Geometry check sheet. Reference: the model listing, model coordinates, mm. Coordinates: 2 decimals unless noted, no trailing zeros. Order: outer loops, then holes, each group sorted by start corner. A loop starts at its lowest first (then second) coordinate and runs counter-clockwise, first axis right, second up. Notation, with made-up numbers: (-13, 53.25) - (3, 53.25) arc R22 ccw to (3, 86.25) - close; hole circle Ø9 at (20, -18.75). An arc over 180 degrees is marked (long way). Use CSV: the item, a comma, the result in double quotes. Start each with the question number.
1) Depth check by flat-ended pin: P1, Ø4, axis at x = 5, y = 6, coming from the +Z side. Enter the tip coordinate at first touch or a pass-through.
2) Sectioned sample at B-B, the plane y = 6. Record the cut outline in (x, z).
3) Sectioned sample at C-C, the plane z = 8.75. Record the cut outline in (x, y).
4) Sectioned sample at D-D, the plane x = 7. Record the cut outline in (y, z), and give its area (3 significant figures).
5) Sectioned sample at A-A, the plane x = 5. Record the cut outline in (y, z), and give its area (3 significant figures).
6) Thickness scan on probe 1 along Y at (x, z) = (5, 2); probe 2 along Y at (x, z) = (5, 9.35); probe 3 along X at (y, z) = (14, 2.25). Record the ranges inside material, lowest first. Write a range as [from, to].
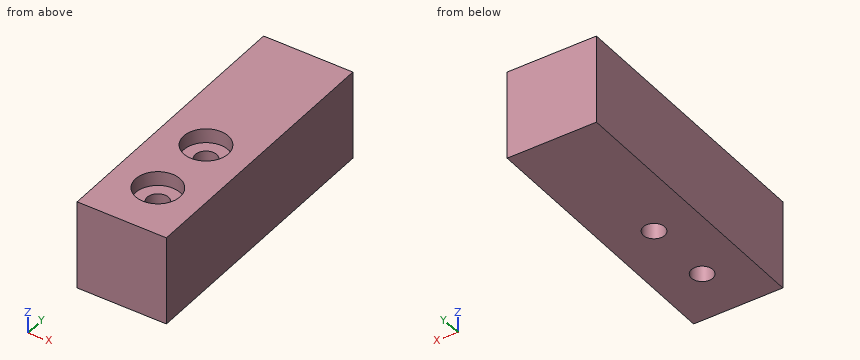
from build123d import *

# Parameters (mm, degrees)
SKETCH1_W                                = 10
SKETCH1_H                                = 31
BOSS_EXTRUDE1_DEPTH                      = 10
CBORE_FOR_M2_PAN_HEAD_SCREW1_D           = 2.4
CBORE_FOR_M2_PAN_HEAD_SCREW1_DEPTH       = 10
CBORE_FOR_M2_PAN_HEAD_SCREW1_CBORE_D     = 5
CBORE_FOR_M2_PAN_HEAD_SCREW1_CBORE_DEPTH = 1.6
CBORE_FOR_M2_PAN_HEAD_SCREW1_TIP         = 0.721032743


with BuildPart() as part:
    # Sketch1 → Boss-Extrude1 (new body)
    with BuildSketch(Plane.XY):
        with Locations((5, 15.5)):
            Rectangle(SKETCH1_W, SKETCH1_H)
    extrude(amount=BOSS_EXTRUDE1_DEPTH)

    # CBORE for M2 Pan Head Screw1
    with Locations(Plane(origin=(5, 14, 10), x_dir=(1, 0, 0), z_dir=(0, 0, 1))):
        with Locations((0, 0), (0, -8)):
            CounterBoreHole(CBORE_FOR_M2_PAN_HEAD_SCREW1_D / 2, CBORE_FOR_M2_PAN_HEAD_SCREW1_CBORE_D / 2, CBORE_FOR_M2_PAN_HEAD_SCREW1_CBORE_DEPTH, depth=CBORE_FOR_M2_PAN_HEAD_SCREW1_DEPTH)
            with Locations((0, 0, -(CBORE_FOR_M2_PAN_HEAD_SCREW1_DEPTH + CBORE_FOR_M2_PAN_HEAD_SCREW1_TIP / 2))):  # 118° drill point
                Cone(0, CBORE_FOR_M2_PAN_HEAD_SCREW1_D / 2, CBORE_FOR_M2_PAN_HEAD_SCREW1_TIP, mode=Mode.SUBTRACT)


solid = part.part
Evaluation:
1,P1,"z = 8.4"
2,outline,"(0, 0) - (3.8, 0) - (3.8, 8.4) - (2.5, 8.4) - (2.5, 10) - (0, 10) - close; (6.2, 0) - (10, 0) - (10, 10) - (7.5, 10) - (7.5, 8.4) - (6.2, 8.4) - close"
3,outline,"(0, 0) - (10, 0) - (10, 31) - (0, 31) - close; hole circle Ø5 at (5, 6); hole circle Ø5 at (5, 14)"
4,outline,"(0, 0) - (31, 0) - (31, 10) - (15.5, 10) - (15.5, 8.4) - (12.5, 8.4) - (12.5, 10) - (7.5, 10) - (7.5, 8.4) - (4.5, 8.4) - (4.5, 10) - (0, 10) - close"
4,area,"300 mm²"
5,outline,"(0, 0) - (4.8, 0) - (4.8, 8.4) - (3.5, 8.4) - (3.5, 10) - (0, 10) - close; (7.2, 0) - (12.8, 0) - (12.8, 8.4) - (11.5, 8.4) - (11.5, 10) - (8.5, 10) - (8.5, 8.4) - (7.2, 8.4) - close; (15.2, 0) - (31, 0) - (31, 10) - (16.5, 10) - (16.5, 8.4) - (15.2, 8.4) - close"
5,area,"254 mm²"
6,probe 1,"[0, 4.8], [7.2, 12.8], [15.2, 31]"
6,probe 2,"[0, 3.5], [8.5, 11.5], [16.5, 31]"
6,probe 3,"[0, 3.8], [6.2, 10]"
